from build123d import *

# Parameters (mm, degrees)
SKETCH1_R               = 1.778
BOSS_EXTRUDE1_DEPTH     = 6.35
SKETCH2_R               = 1.397
CUT_EXTRUDE1_DEPTH      = 100.646453148
FILL_PATTERN1_OUTLINE_R = 1.397
FILL_PATTERN1_DEPTH     = 6.35
SKETCH3_R               = 4.445
CUT_EXTRUDE2_DEPTH      = 3.175


# Read off the part's stored shape, not the designer's step: Fill Pattern1
with BuildPart() as part:
    # Sketch1 → Boss-Extrude1 (new body)
    with BuildSketch(Plane(origin=(0, 0, 0), x_dir=(1, 0, 0), z_dir=(0, 1, 0))):
        with BuildLine():
            Line((23.676158632, 0), (-23.676158632, 0))
            ThreePointArc((-23.676158632, 0), (-25.396043626, 0.058295329), (-27.108034032, 0.232913732))
            Line((-27.108034032, 0.232913732), (-89.75796885, 8.776086661))
            ThreePointArc((-89.75796885, 8.776086661), (-93.68385839, 10.892071009), (-95.25, 15.067858228))
            Line((-95.25, 15.067858228), (-95.25, 22.225))
            ThreePointArc((-95.25, 22.225), (-93.390128061, 26.715128061), (-88.9, 28.575))
            Line((-88.9, 28.575), (-15.24, 28.575))
            ThreePointArc((-15.24, 28.575), (-13.443948776, 27.831051224), (-12.7, 26.035))
            Line((-12.7, 26.035), (-12.7, 17.78))
            ThreePointArc((-12.7, 17.78), (-11.956051224, 15.983948776), (-10.16, 15.24))
            Line((-10.16, 15.24), (10.16, 15.24))
            ThreePointArc((10.16, 15.24), (11.956051224, 15.983948776), (12.7, 17.78))
            Line((12.7, 17.78), (12.7, 26.035))
            ThreePointArc((12.7, 26.035), (13.443948776, 27.831051224), (15.24, 28.575))
            Line((15.24, 28.575), (88.9, 28.575))
            ThreePointArc((88.9, 28.575), (93.390128061, 26.715128061), (95.25, 22.225))
            Line((95.25, 22.225), (95.25, 15.067858228))
            ThreePointArc((95.25, 15.067858228), (93.68385839, 10.892071009), (89.75796885, 8.776086661))
            Line((89.75796885, 8.776086661), (27.108034032, 0.232913732))
            ThreePointArc((27.108034032, 0.232913732), (25.396043626, 0.058295329), (23.676158632, 0))
        make_face()
        with Locations(Location((-60.325, 15.875, 0), (0, 0, 270))):
            Circle(SKETCH1_R, mode=Mode.SUBTRACT)
        with Locations(Location((60.325, 15.875, 0), (0, 0, 90))):
            Circle(SKETCH1_R, mode=Mode.SUBTRACT)
    extrude(amount=BOSS_EXTRUDE1_DEPTH)

    # Sketch2 → Cut-Extrude1 (cut, through all)
    with BuildSketch(Plane(origin=(0, 0, 0), x_dir=(1, 0, 0), z_dir=(0, 1, 0))):
        with Locations(Location((0, 5.08, 0), (0, 0, 270))):
            Circle(SKETCH2_R)
    extrude(amount=CUT_EXTRUDE1_DEPTH, mode=Mode.SUBTRACT)

    # Fill Pattern1 outline → Fill Pattern1 (cut)
    with BuildSketch(Plane(origin=(0, 0, 0), x_dir=(1, 0, 0), z_dir=(0, 1, 0))):
        with Locations((-88.9, 23.557518015)):
            Circle(FILL_PATTERN1_OUTLINE_R)
        with Locations((-85.344, 17.398345343)):
            Circle(FILL_PATTERN1_OUTLINE_R)
        with Locations((-81.788, 23.557518015)):
            Circle(FILL_PATTERN1_OUTLINE_R)
        with Locations((-78.232, 17.398345343)):
            Circle(FILL_PATTERN1_OUTLINE_R)
        with Locations((-74.676, 23.557518015)):
            Circle(FILL_PATTERN1_OUTLINE_R)
        with Locations((-74.676, 11.239172672)):
            Circle(FILL_PATTERN1_OUTLINE_R)
        with Locations((-71.12, 17.398345343)):
            Circle(FILL_PATTERN1_OUTLINE_R)
        with Locations((-67.564, 23.557518015)):
            Circle(FILL_PATTERN1_OUTLINE_R)
        with Locations((-67.564, 11.239172672)):
            Circle(FILL_PATTERN1_OUTLINE_R)
        with Locations((-60.452, 23.557518015)):
            Circle(FILL_PATTERN1_OUTLINE_R)
        with Locations((-53.34, 23.557518015)):
            Circle(FILL_PATTERN1_OUTLINE_R)
        with Locations((-53.34, 11.239172672)):
            Circle(FILL_PATTERN1_OUTLINE_R)
        with Locations((-49.784, 17.398345343)):
            Circle(FILL_PATTERN1_OUTLINE_R)
        with Locations((-46.228, 23.557518015)):
            Circle(FILL_PATTERN1_OUTLINE_R)
        with Locations((-46.228, 11.239172672)):
            Circle(FILL_PATTERN1_OUTLINE_R)
        with Locations((-42.672, 17.398345343)):
            Circle(FILL_PATTERN1_OUTLINE_R)
        with Locations((-39.116, 23.557518015)):
            Circle(FILL_PATTERN1_OUTLINE_R)
        with Locations((-39.116, 11.239172672)):
            Circle(FILL_PATTERN1_OUTLINE_R)
        with Locations((-35.56, 17.398345343)):
            Circle(FILL_PATTERN1_OUTLINE_R)
        with Locations((-32.004, 23.557518015)):
            Circle(FILL_PATTERN1_OUTLINE_R)
        with Locations((-32.004, 11.239172672)):
            Circle(FILL_PATTERN1_OUTLINE_R)
        with Locations((-28.448, 17.398345343)):
            Circle(FILL_PATTERN1_OUTLINE_R)
        with Locations((-24.892, 23.557518015)):
            Circle(FILL_PATTERN1_OUTLINE_R)
        with Locations((-28.448, 5.08)):
            Circle(FILL_PATTERN1_OUTLINE_R)
        with Locations((-24.892, 11.239172672)):
            Circle(FILL_PATTERN1_OUTLINE_R)
        with Locations((-21.336, 17.398345343)):
            Circle(FILL_PATTERN1_OUTLINE_R)
        with Locations((-17.78, 23.557518015)):
            Circle(FILL_PATTERN1_OUTLINE_R)
        with Locations((-21.336, 5.08)):
            Circle(FILL_PATTERN1_OUTLINE_R)
        with Locations((-17.78, 11.239172672)):
            Circle(FILL_PATTERN1_OUTLINE_R)
        with Locations((-14.224, 5.08)):
            Circle(FILL_PATTERN1_OUTLINE_R)
        with Locations((-10.668, 11.239172672)):
            Circle(FILL_PATTERN1_OUTLINE_R)
        with Locations((-7.112, 5.08)):
            Circle(FILL_PATTERN1_OUTLINE_R)
        with Locations((-3.556, 11.239172672)):
            Circle(FILL_PATTERN1_OUTLINE_R)
        with Locations((3.556, 11.239172672)):
            Circle(FILL_PATTERN1_OUTLINE_R)
        with Locations((7.112, 5.08)):
            Circle(FILL_PATTERN1_OUTLINE_R)
        with Locations((10.668, 11.239172672)):
            Circle(FILL_PATTERN1_OUTLINE_R)
        with Locations((17.78, 23.557518015)):
            Circle(FILL_PATTERN1_OUTLINE_R)
        with Locations((14.224, 5.08)):
            Circle(FILL_PATTERN1_OUTLINE_R)
        with Locations((17.78, 11.239172672)):
            Circle(FILL_PATTERN1_OUTLINE_R)
        with Locations((21.336, 17.398345343)):
            Circle(FILL_PATTERN1_OUTLINE_R)
        with Locations((24.892, 23.557518015)):
            Circle(FILL_PATTERN1_OUTLINE_R)
        with Locations((21.336, 5.08)):
            Circle(FILL_PATTERN1_OUTLINE_R)
        with Locations((24.892, 11.239172672)):
            Circle(FILL_PATTERN1_OUTLINE_R)
        with Locations((28.448, 17.398345343)):
            Circle(FILL_PATTERN1_OUTLINE_R)
        with Locations((32.004, 23.557518015)):
            Circle(FILL_PATTERN1_OUTLINE_R)
        with Locations((28.448, 5.08)):
            Circle(FILL_PATTERN1_OUTLINE_R)
        with Locations((32.004, 11.239172672)):
            Circle(FILL_PATTERN1_OUTLINE_R)
        with Locations((35.56, 17.398345343)):
            Circle(FILL_PATTERN1_OUTLINE_R)
        with Locations((39.116, 23.557518015)):
            Circle(FILL_PATTERN1_OUTLINE_R)
        with Locations((39.116, 11.239172672)):
            Circle(FILL_PATTERN1_OUTLINE_R)
        with Locations((42.672, 17.398345343)):
            Circle(FILL_PATTERN1_OUTLINE_R)
        with Locations((46.228, 23.557518015)):
            Circle(FILL_PATTERN1_OUTLINE_R)
        with Locations((46.228, 11.239172672)):
            Circle(FILL_PATTERN1_OUTLINE_R)
        with Locations((49.784, 17.398345343)):
            Circle(FILL_PATTERN1_OUTLINE_R)
        with Locations((53.34, 23.557518015)):
            Circle(FILL_PATTERN1_OUTLINE_R)
        with Locations((53.34, 11.239172672)):
            Circle(FILL_PATTERN1_OUTLINE_R)
        with Locations((60.452, 23.557518015)):
            Circle(FILL_PATTERN1_OUTLINE_R)
        with Locations((67.564, 23.557518015)):
            Circle(FILL_PATTERN1_OUTLINE_R)
        with Locations((67.564, 11.239172672)):
            Circle(FILL_PATTERN1_OUTLINE_R)
        with Locations((71.12, 17.398345343)):
            Circle(FILL_PATTERN1_OUTLINE_R)
        with Locations((74.676, 23.557518015)):
            Circle(FILL_PATTERN1_OUTLINE_R)
        with Locations((74.676, 11.239172672)):
            Circle(FILL_PATTERN1_OUTLINE_R)
        with Locations((78.232, 17.398345343)):
            Circle(FILL_PATTERN1_OUTLINE_R)
        with Locations((81.788, 23.557518015)):
            Circle(FILL_PATTERN1_OUTLINE_R)
        with Locations((85.344, 17.398345343)):
            Circle(FILL_PATTERN1_OUTLINE_R)
        with Locations((88.9, 23.557518015)):
            Circle(FILL_PATTERN1_OUTLINE_R)
    extrude(amount=FILL_PATTERN1_DEPTH, mode=Mode.SUBTRACT)

    # Sketch3 → Cut-Extrude2 (cut)
    with BuildSketch(Plane(origin=(0, 6.35, 0), x_dir=(1, 0, 0), z_dir=(0, 1, 0))):
        with Locations(Location((-60.325, 15.875, 0), (0, 0, 270))):
            Circle(SKETCH3_R)
        with Locations(Location((60.325, 15.875, 0), (0, 0, 270))):
            Circle(SKETCH3_R)
    extrude(amount=-CUT_EXTRUDE2_DEPTH, mode=Mode.SUBTRACT)


solid = part.part
CAD build for the part. Positions are in the model's coordinates, mm. A direction names the side the tool comes from. Give positions to 0.01 mm unless a question says otherwise; leave off trailing zeros. Answer in a Markdown table with one row per item. Add a question column.
Item 1: Band-saw the part on A-A on y = 4.75. Give the number of separate pieces and of enclosed holes in the cut face, then the cut area to 3 significant figures.
Item 2: Tool access for faces 5 (the face through (-62.2, 3.175, -14.9)), 6 (the face through (-93.6, 3.1, -10.8)), 7 (the face through (-12.7, 3, -22)): list every direction of +Z, -Z, +X, -X, +Y, -Y with a clear straight run to the whole face (end or side of a thin tool).
Item 3: Drop flat-ended pins along their axis: P1, Ø2, axis at x = -85.34, z = -17.4, coming from the -Y side; P2, Ø2.5, axis at x = 62, z = -14.5, coming from the +Y side (3 decimals); P3, Ø3, axis at x = 26.5, y = 5.5, coming from the +Z side; P4, Ø3, axis at x = -48, y = 5, coming from the +Z side. Give the stop position or say it passes through.
Item 4: Probe probe 1 along Z at (x, y) = (61.5, 0.75) (3 decimals); probe 2 along X at (y, z) = (5.5, -20.75); probe 3 along Z at (x, y) = (50.5, 4.5) (3 decimals). List the from-to ranges inside material, lowest first.
Item 5: Mould opens along X. For faces 1 (the face through (58, 3.175, -16)), 2 (the face through (93.34, 3.131, -26.764)), 3 (the face through (12.7, 3, -22)), 4 (the face through (1, 0, -14)) say: +X half, -X half, draft (parallel to the pull), parting line (faces both ways), or undercut.
Reply:
| question | item | result |
|---|---|---|
| 1 | separate pieces | 1 |
| 1 | enclosed holes | 69 |
| 1 | area | 3,870 mm^2 |
| 2 | face 5 | +Y |
| 2 | face 6 | +Z, -X, +Y, -Y |
| 2 | face 7 | -Z, +Y, -Y |
| 3 | P1 | passes through |
| 3 | P2 | stops at y = 3.175 |
| 3 | P3 | stops at z = -0.03 |
| 3 | P4 | stops at z = -2.88 |
| 4 | probe 1 | z = -28.575 to -24.481, -22.634 to -17.209, -14.541 to -4.923 |
| 4 | probe 2 | x = -95.25 to -12.7, 12.7 to 95.25 |
| 4 | probe 3 | z = -28.575 to -18.598, -16.199 to -3.423 |
| 5 | face 1 | undercut |
| 5 | face 2 | +X half |
| 5 | face 3 | undercut |
| 5 | face 4 | draft |
